The model under review builds one solid part; all positions refer to its coordinate system, in mm. A direction names the side the tool comes from. Give positions to 0.01 mm unless a question says otherwise; leave off trailing zeros. Order: outer loops, then holes, each group sorted by start corner. A loop starts at its lowest first (then second) coordinate and runs counter-clockwise, first axis right, second up. Notation, with made-up numbers: (2.5, 26.25) - (34.5, 26.25) arc R14 ccw to (34.5, 49.25) - close; hole circle Ø10 at (-28, 33). An arc over 180 degrees is marked (long way). Use a Markdown table: item, result. Add a question column.
```python
from build123d import *

# Parameters (mm, degrees)
SKETCH_1_W          = 55
SKETCH_1_H          = 50
EXTRUDE_1_DEPTH     = 2
SKETCH_2_W          = 2.016430074
SKETCH_2_H          = 50
EXTRUDE_2_DEPTH     = 10
SKETCH_4_W          = 10
SKETCH_4_H          = 2
SKETCH_4_W_2        = 2
SKETCH_4_H_2        = 10
EXTRUDE_3_DEPTH     = 53
SKETCH_5_W          = 12
SKETCH_5_H          = 6
CUT_EXTRUDE_1_DEPTH = 40
SKETCH_6_W          = 46
SKETCH_6_H          = 6
CUT_EXTRUDE_3_DEPTH = 2
SKETCH_7_W          = 3
SKETCH_7_H          = 50
EXTRUDE_4_DEPTH     = 14
SKETCH_8_W          = 50
SKETCH_8_H          = 2
EXTRUDE_5_DEPTH     = 10


with BuildPart() as part:
    # 草图1 → 凸台-拉伸1 (new body)
    with BuildSketch(Plane(origin=(0, 0, 0), x_dir=(1, 0, 0), z_dir=(0, 1, 0))):
        with Locations((-15.105645182, 3.897173973)):
            Rectangle(SKETCH_1_W, SKETCH_1_H)
    extrude(amount=EXTRUDE_1_DEPTH)

    # 草图2 → 凸台-拉伸2 (add)
    with BuildSketch(Plane(origin=(0, 2, 0), x_dir=(1, 0, 0), z_dir=(0, 1, 0))):
        with Locations((11.386139781, 3.897173973)):
            Rectangle(SKETCH_2_W, SKETCH_2_H)
    extrude(amount=EXTRUDE_2_DEPTH)

    # 草图4 → 凸台-拉伸3 (add)
    with BuildSketch(Plane.ZY.offset(-10.377924744)):
        with Locations((-14.897173973, 11)):
            Rectangle(SKETCH_4_W, SKETCH_4_H)
        Polygon((-28.897173973, 12), (-26.897173973, 12), (-24.897173973, 12), (-24.897173973, 10), (-26.897173973, 10), (-26.897173973, 2), (-28.897173973, 2), align=None)
        Polygon((-2.897173973, 10), (-2.897173973, 2), (-0.897173973, 2), (-0.897173973, 12), (-2.897173973, 12), (-5.725601098, 12), (-5.725601098, 10), align=None)
        with Locations((9.102826027, 11)):
            Rectangle(SKETCH_4_W, SKETCH_4_H)
        with Locations((20.102826027, 7)):
            Rectangle(SKETCH_4_W_2, SKETCH_4_H_2)
    extrude(amount=EXTRUDE_3_DEPTH)

    # 草图5 → 切除-拉伸1 (cut)
    with BuildSketch(Plane(origin=(12.394354818, 0, 0), x_dir=(0, 0, -1), z_dir=(1, 0, 0))):
        with Locations((14.897173973, 6)):
            Rectangle(SKETCH_5_W, SKETCH_5_H)
    extrude(amount=-CUT_EXTRUDE_1_DEPTH, mode=Mode.SUBTRACT)

    # 草图6 → 切除-拉伸3 (cut)
    with BuildSketch(Plane(origin=(0, 12, 0), x_dir=(1, 0, 0), z_dir=(0, 1, 0))):
        with Locations((-19.622075256, 12.897173973)):
            Rectangle(SKETCH_6_W, SKETCH_6_H)
    extrude(amount=-CUT_EXTRUDE_3_DEPTH, mode=Mode.SUBTRACT)

    # 草图7 → 凸台-拉伸4 (add)
    with BuildSketch(Plane.XZ):
        with Locations((10.894354818, -3.897173973)):
            Rectangle(SKETCH_7_W, SKETCH_7_H)
    extrude(amount=EXTRUDE_4_DEPTH)

    # 草图8 → 凸台-拉伸5 (add)
    with BuildSketch(Plane.ZY.offset(-9.394354818)):
        with Locations((-3.897173973, -13)):
            Rectangle(SKETCH_8_W, SKETCH_8_H)
    extrude(amount=EXTRUDE_5_DEPTH)


solid = part.part
```
Q1. Draft analysis for pull direction Z (two halves, no side actions). For faces 6 (the flat face through (-16, 2, 9)), 7 (the flat face through (-42.622, 8, -2)), 8 (the flat face through (-9, 5, -28.897)), state which applies: pulls with the +Z half, pulls with the -Z half, needs draft (parallel to the pull), parting line crosses it, or undercut.
Q2. Wall thickness on probe 1 along Y at (x, z) = (6, -25); probe 2 along Z at (x, y) = (-21, 10.5); probe 3 along Z at (x, y) = (-30.5, 7.5): over which ranges is each line inside the solid? List them lowest first.
Q3. We need section B-B (x = -31). Write out the cut boundary in (y, z), plus the area to 3 significant figures.
Q4. We need section A-A (y = 5.25). Write out the cut boundary in (x, z).
Q5. Machinability: for faces 1 (the flat face through (-42.622, 7, 20)), 2 (the flat face through (11, 6, -8.897)), 3 (the flat face through (-16, 11, 4.103)), 4 (the flat face through (-16, 6, -26.897)), 5 (the flat face through (-0.606, -13, -4)), which of the approach directions +Z, -Z, +X, -X, +Y, -Y give a long, thin tool a straight path to every point of the face, cutting with its end or side? Answer none if there is none.
Q6. We need section D-D (y = -11.25). Write out the cut boundary in (x, z), plus the area to 3 significant figures.
Q7. Clearance check with flat-ended pins moving along their axes: P1, Ø0.6, axis at x = -3, z = -26.5, coming from the -Y side; P2, Ø1.5, axis at x = -4.5, z = 15.5, coming from the +Y side; P3, Ø1, axis at y = -13, z = -12.5, coming from the -X side. State where each tip first meets the part, or that it passes through.
Q8. We need section C-C (z = 11). Write out the cut boundary in (x, y), plus the area to 3 significant figures.
Here are the results:
| question | item | result |
|---|---|---|
| 1 | face 6 | undercut |
| 1 | face 7 | needs draft |
| 1 | face 8 | pulls with the -Z half |
| 2 | probe 1 | -14 to -12, 0 to 2, 10 to 12 |
| 2 | probe 2 | -28.9 to -24.9, -19.9 to -15.9, -5.73 to -0.9, 4.1 to 14.1, 19.1 to 21.1 |
| 2 | probe 3 | -28.9 to -26.9, -2.9 to -0.9, 19.1 to 21.1 |
| 3 | outline | (0, -28.9) - (12, -28.9) - (12, -24.9) - (10, -24.9) - (10, -26.9) - (2, -26.9) - (2, -2.9) - (10, -2.9) - (10, -5.73) - (12, -5.73) - (12, -0.9) - (2, -0.9) - (2, 19.1) - (12, 19.1) - (12, 21.1) - (0, 21.1) - close; (10, -19.9) - (12, -19.9) - (12, -15.9) - (10, -15.9) - close; (10, 4.1) - (12, 4.1) - (12, 14.1) - (10, 14.1) - close |
| 3 | area | 198 mm2 |
| 4 | outline | (-42.62, -28.9) - (12.39, -28.9) - (12.39, -20.9) - (10.38, -20.9) - (10.38, -26.9) - (-42.62, -26.9) - close; (-42.62, -2.9) - (10.38, -2.9) - (10.38, -8.9) - (12.39, -8.9) - (12.39, 21.1) - (-42.62, 21.1) - (-42.62, 19.1) - (10.38, 19.1) - (10.38, -0.9) - (-42.62, -0.9) - close |
| 5 | face 1 | +Z, -Z, -X, +Y, -Y |
| 5 | face 2 | +X, -X |
| 5 | face 3 | -X, +Y |
| 5 | face 4 | -X |
| 5 | face 5 | +Z, -Z, -X, -Y |
| 6 | outline | (9.39, -28.9) - (12.39, -28.9) - (12.39, 21.1) - (9.39, 21.1) - close |
| 6 | area | 150 mm2 |
| 7 | P1 | y = 0 |
| 7 | P2 | y = 2 |
| 7 | P3 | x = -0.61 |
| 8 | outline | (-42.62, 10) - (10.38, 10) - (10.38, 2) - (-42.61, 2) - (-42.61, 0) - (9.39, 0) - (9.39, -12) - (-0.61, -12) - (-0.61, -14) - (12.39, -14) - (12.39, 12) - (-42.62, 12) - close |
| 8 | area | 298 mm2 |
